from build123d import *

# Parameters (mm, degrees)
SKETCH1_R                      = 50.8
SKETCH1_R_2                    = 47.625
EXTRUDE_THIN1_DEPTH            = 301.625
CUT_EXTRUDE1_REACH             = 52.8
SKETCH2_W                      = 38.1
SKETCH2_H                      = 31.75
CUT_EXTRUDE2_REACH             = 52.8
SKETCH3_R                      = 2.54
CUT_EXTRUDE2_DIRECTION_2_REACH = 52.8
CUT_EXTRUDE3_REACH             = 52.8
SKETCH4_R                      = 2.54


with BuildPart() as part:
    # Sketch1 → Extrude-Thin1 (new body)
    with BuildSketch(Plane(origin=(0, 0, 0), x_dir=(1, 0, 0), z_dir=(0, 1, 0))):
        Circle(SKETCH1_R)
        Circle(SKETCH1_R_2, mode=Mode.SUBTRACT)
    extrude(amount=EXTRUDE_THIN1_DEPTH)

    # Sketch2 → Cut-Extrude1 (cut, up to next)
    with BuildSketch(Plane.XY, mode=Mode.PRIVATE) as cut_extrude1_sk1:
        with Locations((0, 301.625)):
            Rectangle(SKETCH2_W, SKETCH2_H)
    cut_extrude1_tool1 = extrude(cut_extrude1_sk1.sketch, amount=-CUT_EXTRUDE1_REACH, mode=Mode.PRIVATE) & part.part
    add(cut_extrude1_tool1.solids().sort_by_distance((0, 301.625, 0))[0], mode=Mode.SUBTRACT)

    # Sketch3 → Cut-Extrude2 (cut, up to next)
    with BuildSketch(Plane(origin=(0, 0, 0), x_dir=(0, 0, -1), z_dir=(1, 0, 0)), mode=Mode.PRIVATE) as cut_extrude2_sk1:
        with Locations((0, 50.8)):
            Circle(SKETCH3_R)
    cut_extrude2_tool1 = extrude(cut_extrude2_sk1.sketch, amount=-CUT_EXTRUDE2_REACH, mode=Mode.PRIVATE) & part.part
    add(cut_extrude2_tool1.solids().sort_by_distance((0, 50.8, 0))[0], mode=Mode.SUBTRACT)

    # Sketch3 → Cut-Extrude2 direction 2 (cut, up to next)
    with BuildSketch(Plane(origin=(0, 0, 0), x_dir=(0, 0, -1), z_dir=(1, 0, 0)), mode=Mode.PRIVATE) as cut_extrude2_direction_2_sk1:
        with Locations((0, 50.8)):
            Circle(SKETCH3_R)
    cut_extrude2_direction_2_tool1 = extrude(cut_extrude2_direction_2_sk1.sketch, amount=CUT_EXTRUDE2_DIRECTION_2_REACH, mode=Mode.PRIVATE) & part.part
    add(cut_extrude2_direction_2_tool1.solids().sort_by_distance((0, 50.8, 0))[0], mode=Mode.SUBTRACT)

    # Sketch4 → Cut-Extrude3 (cut, up to next)
    with BuildSketch(Plane(origin=(0, 0, 0), x_dir=(0, 0, -1), z_dir=(1, 0, 0)), mode=Mode.PRIVATE) as cut_extrude3_sk1:
        with Locations((0, 203.2)):
            Circle(SKETCH4_R)
    cut_extrude3_tool1 = extrude(cut_extrude3_sk1.sketch, amount=-CUT_EXTRUDE3_REACH, mode=Mode.PRIVATE) & part.part
    add(cut_extrude3_tool1.solids().sort_by_distance((0, 203.2, 0))[0], mode=Mode.SUBTRACT)


solid = part.part
Check sheet for the modelled part. Datum: model origin and axes. Units: mm. A direction names the side the tool comes from. Round coordinates to 2 decimals unless told otherwise and drop trailing zeros. Order: outer loops, then holes, each group sorted by start corner. A loop starts at its lowest first (then second) coordinate and runs counter-clockwise, first axis right, second up.
(1) Scan lines: probe 1 along Y at (x, z) = (-49.6, 0) (3 decimals); probe 2 along Y at (x, z) = (49.6, 0) (3 decimals); probe 3 along Z at (x, y) = (0.5, 198). Record each from-to range of solid material in increasing order.
(2) Cross-section at A-A, the plane x = 0. Enter the section's corners in (y, z) (3 decimals).
(3) Cross-section at B-B, the plane z = 30. Enter the section's corners in (x, y) (3 decimals), and give its area (3 significant figures).
(4) Go/stop test with flat-tipped pins: P1, Ø12, axis at x = 28, z = 34.5, coming from the -Y side; P2, Ø1, axis at y = 82.5, z = -16, coming from the +X side; P3, Ø5, axis at y = 163.5, z = 13, coming from the -X side; P4, Ø5, axis at x = 1.5, y = 230.5, coming from the +Z side. Record where each tip stops, or that it passes through.
(5) Cross-section at C-C, the plane y = 42. Enter the section's corners in (x, z) (3 decimals), and give its area (3 significant figures).
(6) Draft check along Z on faces 4 (the cylindrical face through (-49.16, 48.32, 0.55)), 5 (the cylindrical face through (-11.012, 148.701, 49.592)), 6 (the flat face through (0, 301.625, 49)). Enter one of: pulls with the +Z half, pulls with the -Z half, needs draft (parallel to the pull), parting line crosses it, or undercut.
(7) Access from +Z, -Z, +X, -X, +Y, -Y to the whole of each face (thin tool, end or side, straight path). Record for faces 1 (the cylindrical face through (-37.794, 148.701, 28.979)), 2 (the cylindrical face through (-49.16, 200.72, 0.55)), 3 (the flat face through (0, 285.75, -48)).
Check sheet entries:
1. probe 1: y = 0 to 48.26, 53.34 to 200.66, 205.74 to 301.625
1. probe 2: y = 0 to 48.26, 53.34 to 301.625
1. probe 3: z = -50.8 to -47.62, 47.62 to 50.8
2. outline: (0, -50.8) - (285.75, -50.8) - (285.75, -47.625) - (0, -47.625) - close; (0, 47.625) - (301.625, 47.625) - (301.625, 50.8) - (0, 50.8) - close
3. outline: (-40.996, 0) - (-36.988, 0) - (-36.988, 301.625) - (-40.996, 301.625) - close; (36.988, 0) - (40.996, 0) - (40.996, 301.625) - (36.988, 301.625) - close
3. area: 2,420 mm2
4. P1: stops at y = 0
4. P2: stops at x = 48.38
4. P3: stops at x = -49.7
4. P4: stops at z = 50.8
5. outline: circle Ø101.6 at (0, 0); hole circle Ø95.25 at (0, 0)
5. area: 982 mm2
6. face 4: undercut
6. face 5: parting line crosses it
6. face 6: needs draft
7. face 1: +Y, -Y
7. face 2: -X
7. face 3: -Z, +Y
